from build123d import *

# Parameters (mm, degrees)
F0_W     = 25.4
F0_H     = 25.4
F1_DEPTH = 10
F3_DEPTH = 7.5
F4_R     = 6.35
F5_SIZE  = 2.5


with BuildPart() as f1:
    # F0 (on Top) → F1 (new body)
    with BuildSketch(Plane.XY):
        Rectangle(F0_W, F0_H)
        Polygon((-2.066667, -3.970835), (-2.066667, -7.723612), (-5.316667, -9.6), (-8.566667, -7.723612), (-8.566667, -3.970835), (-5.316667, -2.094447), align=None, mode=Mode.SUBTRACT)
        Polygon((5.316667, -2.094447), (8.566667, -3.970835), (8.566667, -7.723612), (5.316667, -9.6), (2.066667, -7.723612), (2.066667, -3.970835), align=None, mode=Mode.SUBTRACT)
        Polygon((-5.316667, 9.6), (-2.066667, 7.723612), (-2.066667, 3.970835), (-5.316667, 2.094447), (-8.566667, 3.970835), (-8.566667, 7.723612), align=None, mode=Mode.SUBTRACT)
        Polygon((2.066667, 3.970835), (2.066667, 7.723612), (5.316667, 9.6), (8.566667, 7.723612), (8.566667, 3.970835), (5.316667, 2.094447), align=None, mode=Mode.SUBTRACT)
        Polygon((-5.316667, -9.6), (-2.066667, -7.723612), (-2.066667, -3.970835), (-5.316667, -2.094447), (-8.566667, -3.970835), (-8.566667, -7.723612), align=None)
        Polygon((5.316667, 9.6), (2.066667, 7.723612), (2.066667, 3.970835), (5.316667, 2.094447), (8.566667, 3.970835), (8.566667, 7.723612), align=None)
        Polygon((8.566667, -7.723612), (8.566667, -3.970835), (5.316667, -2.094447), (2.066667, -3.970835), (2.066667, -7.723612), (5.316667, -9.6), align=None)
        Polygon((-2.066667, 3.970835), (-2.066667, 7.723612), (-5.316667, 9.6), (-8.566667, 7.723612), (-8.566667, 3.970835), (-5.316667, 2.094447), align=None)
    extrude(amount=F1_DEPTH)

    # F2 (on face) → F3 (cut)
    with BuildSketch(Plane.XY.offset(10)):
        Polygon((-5.316667, 9.6), (-8.566667, 7.723612), (-8.566667, 3.970835), (-5.316667, 2.094447), (-2.066667, 3.970835), (-2.066667, 7.723612), align=None)
        Polygon((2.066667, 3.970835), (5.316667, 2.094447), (8.566667, 3.970835), (8.566667, 7.723612), (5.316667, 9.6), (2.066667, 7.723612), align=None)
        Polygon((5.316667, -2.094447), (2.066667, -3.970835), (2.066667, -7.723612), (5.316667, -9.6), (8.566667, -7.723612), (8.566667, -3.970835), align=None)
        Polygon((-5.316667, -2.094447), (-8.566667, -3.970835), (-8.566667, -7.723612), (-5.316667, -9.6), (-2.066667, -7.723612), (-2.066667, -3.970835), align=None)
    extrude(amount=-F3_DEPTH, mode=Mode.SUBTRACT)

    # F4
    f4_edges = [f1.edges().sort_by_distance(p)[0] for p in [
        (-12.7, -12.7, 5),
        (12.7, -12.7, 5),
        (12.7, 12.7, 5),
        (-12.7, 12.7, 5),
    ]]
    fillet(f4_edges, radius=F4_R)

    # F5
    f5_edges = [f1.edges().sort_by_distance(p)[0] for p in [
        (-12.7, 0, 10),
        (0, -12.7, 10),
        (12.7, 0, 10),
        (0, 12.7, 10),
    ]]
    chamfer(f5_edges, length=F5_SIZE)


solid = f1.part
The listing builds one solid part. Answer for the finished solid, in the listing's coordinates (mm). A direction names the side the tool comes from. Round coordinates to 2 decimals unless told otherwise and drop trailing zeros. Loops run counter-clockwise (first coordinate to the right, second up) from the corner with the lowest first, then second, coordinate; pieces in that order, holes last. Notation, with made-up numbers: M 50,88.5 L 74,88.5 A31 cw 74,126.5 Z; hole C -27,-26 d3. An arc over 180 degrees is marked long. Return JSON: item names as keys, results as strings.
Q1. Find section B-B, the plane z = 1. Determine the outline of the cut face in (x, y), plus the area to 3 significant figures.
Results list:
{"outline": "M -12.7,-6.35 A6.35 ccw -6.35,-12.7 L 6.35,-12.7 A6.35 ccw 12.7,-6.35 L 12.7,6.35 A6.35 ccw 6.35,12.7 L -6.35,12.7 A6.35 ccw -12.7,6.35 Z", "area": "611 mm2"}
Q2. Which of the six approach directions +Z, -Z, +X, -X, +Y, -Y give full straight-line access (tool end or side, diameter ignored) to faces 4 (the face through (-9.78, 9.71, 9.05)), 5 (the face through (6.96, 8.65, 6.3))?
Results list:
{"face 4": "+Z, -X, +Y", "face 5": "+Z"}
Q3. Find section A-A, the plane z = 8. State how many separate pieces and enclosed holes the cut face has, plus the area to 3 significant figures.
Results list:
{"separate pieces": "1", "enclosed holes": "4", "area": "420 mm2"}
Q4. Each of these flat-tipped pins is pushed along its axis until it touches: pin 1 Ø5 at (x, z) = (-7, 3.5) entering from +Y; pin 2 Ø2 at (y, z) = (-3.5, 9) entering from +X; pin 3 Ø2 at (x, y) = (-5, 7.5) entering from +Z. Where does it stop, or does it pass through?
Results list:
{"pin 1": "stops at y = 12.7", "pin 2": "stops at x = 12.2", "pin 3": "stops at z = 2.5"}
Q5. Find section C-C, the plane x = -3.25. Determine the outline of the cut face in (y, z).
Results list:
{"outline": "M -12.7,0 L 12.7,0 L 12.7,7.5 L 10.2,10 L 8.41,10 L 8.41,2.5 L 3.29,2.5 L 3.29,10 L -3.29,10 L -3.29,2.5 L -8.41,2.5 L -8.41,10 L -10.2,10 L -12.7,7.5 Z"}
Q6. The mould has two halves that part along Y. Classify faces 1 (the face through (-10.89, 10.79, 3.8)), 2 (the face through (2.067, -6, 6)), 3 (the face through (11.4, 0.1, 8.8)): released by +Y, released by -Y, zero draft, split by the parting line, or undercut.
Results list:
{"face 1": "released by +Y", "face 2": "undercut", "face 3": "zero draft"}
Q7. Find section D-D, the plane y = -5.75. Determine the outline of the cut face in (x, z).
Results list:
{"outline": "M -12.7,0 L 12.7,0 L 12.7,7.5 L 10.2,10 L 8.57,10 L 8.57,2.5 L 2.07,2.5 L 2.07,10 L -2.07,10 L -2.07,2.5 L -8.57,2.5 L -8.57,10 L -10.2,10 L -12.7,7.5 Z"}
Q8. Find the intervals of material crossed by line 1 along X through (y, z) = (-4.25, 4.25); line 2 along X through (y, z) = (9.5, 3.25); line 3 along Y through (x, z) = (2.5, 6.5), in increasing order. Write a range as from..to.
Results list:
{"line 1": "x = -12.7..-8.57, -2.07..2.07, 8.57..12.7", "line 2": "x = -11.86..-5.49, -5.14..5.14, 5.49..11.86", "line 3": "y = -12.7..-7.97, -3.72..3.72, 7.97..12.7"}
